For this review, take the finished solid that the model builds, in its own axes (mm). A direction names the side the tool comes from. Give positions to 0.01 mm unless a question says otherwise; leave off trailing zeros. Order: outer loops, then holes, each group sorted by start corner. A loop starts at its lowest first (then second) coordinate and runs counter-clockwise, first axis right, second up. Notation, with made-up numbers: (11, -18.5) -> (60, -18.5) arc R20 ccw to (60, 5.5) -> close; hole circle Ø2 at (-23.75, 62). An arc over 180 degrees is marked (long way). Use CSV: the item, a comma, the result in double quotes. Start each with the question number.
```python
from build123d import *

# Parameters (mm, degrees)
SKETCH1_R             = 14.2875
BOSS_EXTRUDE1_DEPTH   = 25.4
SKETCH3_R             = 11.1125
CUT_EXTRUDE1_DEPTH    = 7.14375
CUT_EXTRUDE2_DEPTH    = 18.25625
CUT_EXTRUDE3_START    = -11.90625
SKETCH5_R             = 11.1125
CUT_EXTRUDE3_DEPTH    = 11.90625
F_4_40_TAPPED_HOLE1_D = 2.2606
CIRPATTERN1_COUNT     = 4
SKETCH8_R             = 3.1496
CUT_EXTRUDE6_DEPTH    = 33.456514177


with BuildPart() as part:
    # Sketch1 → Boss-Extrude1 (new body)
    with BuildSketch(Plane(origin=(0, 0, 0), x_dir=(1, 0, 0), z_dir=(0, 1, 0))):
        with Locations(Location((0, 0, 0), (0, 0, 270))):
            Circle(SKETCH1_R)
    extrude(amount=BOSS_EXTRUDE1_DEPTH)

    # Sketch3 → Cut-Extrude1 (cut)
    with BuildSketch(Plane.XZ):
        with Locations(Location((0, 0, 0), (0, 0, 270))):
            Circle(SKETCH3_R)
    extrude(amount=-CUT_EXTRUDE1_DEPTH, mode=Mode.SUBTRACT)

    # Sketch4 → Cut-Extrude2 (cut)
    with BuildSketch(Plane(origin=(0, 25.4, 0), x_dir=(1, 0, 0), z_dir=(0, 1, 0))):
        with BuildLine():
            Line((-1.5875, 7.9375), (1.5875, 7.9375))
            ThreePointArc((1.5875, 7.9375), (6.077628061, 6.077628061), (7.9375, 1.5875))
            Line((7.9375, 1.5875), (7.9375, -1.5875))
            ThreePointArc((7.9375, -1.5875), (6.077628061, -6.077628061), (1.5875, -7.9375))
            Line((1.5875, -7.9375), (-1.5875, -7.9375))
            ThreePointArc((-1.5875, -7.9375), (-6.077628061, -6.077628061), (-7.9375, -1.5875))
            Line((-7.9375, -1.5875), (-7.9375, 1.5875))
            ThreePointArc((-7.9375, 1.5875), (-6.077628061, 6.077628061), (-1.5875, 7.9375))
        make_face()
    extrude(amount=-CUT_EXTRUDE2_DEPTH, mode=Mode.SUBTRACT)

    # Sketch5 → Cut-Extrude3 (cut)
    with BuildSketch(Plane(origin=(0, 25.4, 0), x_dir=(1, 0, 0), z_dir=(0, 1, 0)).offset(CUT_EXTRUDE3_START)):
        with Locations(Location((0, 0, 0), (0, 0, 90))):
            Circle(SKETCH5_R)
    extrude(amount=CUT_EXTRUDE3_DEPTH, mode=Mode.SUBTRACT)

    # 4-40 Tapped Hole1 (through all)
    with Locations(Plane(origin=(0, 13.49375, 0), x_dir=(-1, 0, 0), z_dir=(0, 1, 0))):
        with Locations((0, -9.525)):
            f_4_40_tapped_hole1 = Hole(F_4_40_TAPPED_HOLE1_D / 2)

    # CirPattern1: 4-40 Tapped Hole1 ×4 about axis
    cirpattern1_axis = Axis((0, 0, 0), (0, 1, 0))
    for i in range(1, CIRPATTERN1_COUNT):
        add(f_4_40_tapped_hole1.rotate(cirpattern1_axis, i * 360 / CIRPATTERN1_COUNT), mode=Mode.SUBTRACT)

    # Sketch8 → Cut-Extrude6 (cut, through all)
    with BuildSketch(Plane(origin=(0, 0, 0), x_dir=(-0.7071067811865488, 0, -0.7071067811865464), z_dir=(0.7071067811865464, 0, -0.7071067811865488))):
        with Locations((0, 10.31875)):
            Circle(SKETCH8_R)
    extrude(amount=-CUT_EXTRUDE6_DEPTH, mode=Mode.SUBTRACT)


solid = part.part
```
1. Consider section C-C (x = 6.25). State the section outline as (y, z) points.
2. To check wall thickness, follow L1, parallel to X at y = 11.75, z = 0; L2, parallel to X at y = 22.75, z = 0.25; L3, parallel to Y at x = -10.25, z = 1.5. State the ranges of each line that lie inside material, in increasing order. Write a range as [from, to].
3. Clearance check with flat-ended pins moving along their axes: P1, Ø6, axis at x = 8, z = 0, coming from the +Y side; P2, Ø1, axis at x = -2.5, z = 9, coming from the -Y side; P3, Ø3, axis at y = 3.5, z = 10, coming from the -X side; P4, Ø1.8, axis at x = 0, z = -9.525, coming from the +Y side. State where each tip first meets the part, or that it passes through.
4. Consider section B-B (x = 0). State the section outline as (y, z) points, plus the area to 3 significant figures.
5. Consider section D-D (y = 13). State how many separate pieces and enclosed holes the cut face has, plus the area to 3 significant figures.
6. For faces 4 (the face through (-9.37, 19.364, -5.974)), 5 (the face through (8.3, 7.144, -0.8)), 6 (the face through (-3.16, 9.66, 7.74)), list the 3-axis set-ups (+Z, -Z, +X, -X, +Y, -Y) from which the entire face can be reached by the end or side of a thin tool; tool diameter is ignored.
7. Consider section A-A (z = 0). State the section outline as (x, y) points.
8. Draft analysis for pull direction Z (two halves, no side actions). For faces 1 (the face through (0.628, 12.522, -14.274)), 2 (the face through (-7.938, 10, 0)), 3 (the face through (-7, 25.4, -9)), state which applies: +Z half, -Z half, draft (parallel to the pull), parting line (faces both ways), or undercut.
Answer list:
1,outline,"(0, -12.85) -> (25.4, -12.85) -> (25.4, -9.19) -> (13.49, -9.19) -> (13.49, -5.9) -> (7.14, -5.9) -> (7.14, -9.19) -> (0, -9.19) -> close; (0, 9.19) -> (7.14, 9.19) -> (7.14, 5.9) -> (13.49, 5.9) -> (13.49, 9.19) -> (25.4, 9.19) -> (25.4, 12.85) -> (0, 12.85) -> close"
2,L1,"[-14.29, -10.66], [-8.39, -7.94], [7.94, 8.39], [10.66, 14.29]"
2,L2,"[-14.29, -11.11], [11.11, 14.29]"
2,L3,"[7.14, 13.49]"
3,P1,"y = 13.49"
3,P2,"y = 7.14"
3,P3,"x = -11.48"
3,P4,"through"
4,outline,"(0, -14.29) -> (25.4, -14.29) -> (25.4, -11.11) -> (13.49, -11.11) -> (13.49, -10.66) -> (7.14, -10.66) -> (7.14, -11.11) -> (0, -11.11) -> close; (0, 11.11) -> (7.14, 11.11) -> (7.14, 10.66) -> (13.49, 10.66) -> (13.49, 11.11) -> (25.4, 11.11) -> (25.4, 14.29) -> (0, 14.29) -> close; (7.14, -8.39) -> (13.49, -8.39) -> (13.49, -7.94) -> (7.14, -7.94) -> close; (7.14, 7.94) -> (13.49, 7.94) -> (13.49, 8.39) -> (7.14, 8.39) -> close"
4,area,"173 mm2"
5,separate pieces,"1"
5,enclosed holes,"4"
5,area,"389 mm2"
6,face 4,"+Y"
6,face 5,"-Y"
6,face 6,"+Y, -Y"
7,outline,"(-14.29, 0) -> (-11.11, 0) -> (-11.11, 7.14) -> (-10.66, 7.14) -> (-10.66, 13.49) -> (-11.11, 13.49) -> (-11.11, 25.4) -> (-14.29, 25.4) -> close; (-8.39, 7.14) -> (-7.94, 7.14) -> (-7.94, 13.49) -> (-8.39, 13.49) -> close; (7.94, 7.14) -> (8.39, 7.14) -> (8.39, 13.49) -> (7.94, 13.49) -> close; (10.66, 7.14) -> (11.11, 7.14) -> (11.11, 0) -> (14.29, 0) -> (14.29, 25.4) -> (11.11, 25.4) -> (11.11, 13.49) -> (10.66, 13.49) -> close"
8,face 1,"parting line"
8,face 2,"undercut"
8,face 3,"draft"
